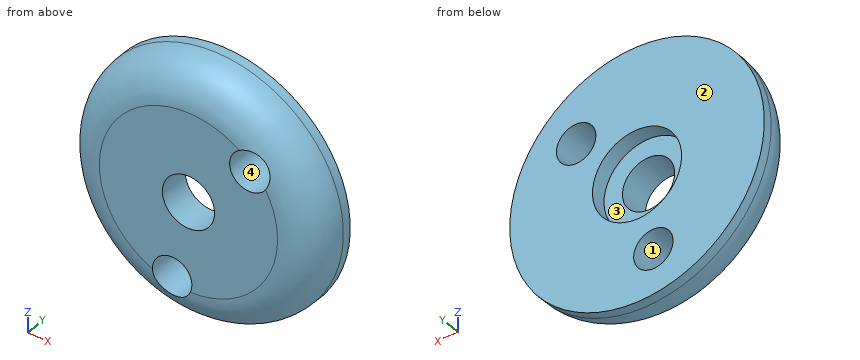
```python
from build123d import *

# Parameters (mm, degrees)
BOSS_EXTRUDE1_DEPTH        = 3
BOSS_EXTRUDE1_DEPTH_BACK   = 10
SKETCH1_R                  = 10
SKETCH4_R                  = 1.5
HOLE_DEPTH                 = 20.973741561
HOLECIR_COUNT              = 5
SKETCH6_R                  = 3.5
BEARINGHOLE_DEPTH          = 2.5
SKETCH7_R                  = 2.05
SHAFTHOLE_DEPTH            = 17.248076982
F_3_1_3_1_DIAMETER_HOLE1_D = 3.1
FILLET2_R                  = 3
SKETCH11_R                 = 10
CUT_EXTRUDE1_DEPTH         = 10


with BuildPart() as part:
    # Sketch1 → Boss-Extrude1 (new, two sides: drawn at the far end of the back side and taken through both)
    with BuildSketch(Plane(origin=(0, 0, 0), x_dir=(1, 0, 0), z_dir=(0, 1, 0)).offset(-BOSS_EXTRUDE1_DEPTH_BACK)):
        with Locations(Location((0, 0, 0), (0, 0, 270))):
            Circle(SKETCH1_R)
    extrude(amount=BOSS_EXTRUDE1_DEPTH + BOSS_EXTRUDE1_DEPTH_BACK)

    # Sketch4 → hole (cut, through all)
    with BuildSketch(Plane(origin=(-3.352872105, -1.093066116, 1.887711608), x_dir=(-0.4486862613641547, -0.14627571033740308, -0.8816371449912632), z_dir=(0.8382180262940947, 0.2732665289126682, -0.47192790187872385))):
        with Locations(Location((0, 0, 0), (0, 0, 8.746528197))):
            Circle(SKETCH4_R)
    hole = extrude(amount=-HOLE_DEPTH, mode=Mode.SUBTRACT)

    # holecir: hole ×5 about axis
    holecir_axis = Axis((0, 0, 0), (0, 1, 0))
    for i in range(1, HOLECIR_COUNT):
        add(hole.rotate(holecir_axis, i * 360 / HOLECIR_COUNT), mode=Mode.SUBTRACT)

    # Sketch6 → bearinghole (cut)
    with BuildSketch(Plane(origin=(0, -5, 0), x_dir=(-1, 0, 0), z_dir=(0, -1, 0))):
        with Locations(Location((0, 0, 0), (0, 0, 90))):
            Circle(SKETCH6_R)
    extrude(amount=BEARINGHOLE_DEPTH, mode=Mode.SUBTRACT)

    # Sketch7 → shafthole (cut, through all)
    with BuildSketch(Plane(origin=(0, -5, 0), x_dir=(-1, 0, 0), z_dir=(0, -1, 0))):
        with Locations(Location((0, 0, 0), (0, 0, 90))):
            Circle(SKETCH7_R)
    extrude(amount=SHAFTHOLE_DEPTH, mode=Mode.SUBTRACT)

    # Ø3.1 (3.1) Diameter Hole1 (through all)
    with Locations(Plane(origin=(0, 3, 0), x_dir=(1, 0, 0), z_dir=(0, 1, 0))):
        with Locations((-1.282558474, 6.372208703), (4.783101903, -4.401356176)):
            Hole(F_3_1_3_1_DIAMETER_HOLE1_D / 2)

    # Fillet2
    # the kernel refuses this fillet: 3 mm, written as the material it takes off along each edge
    with BuildSketch(Plane(origin=(0, 3, 0), x_dir=(0, 0, 1), z_dir=(-1, 0, 0))) as fillet2_piece_1:
        with BuildLine():
            CenterArc((10 - FILLET2_R, -FILLET2_R), FILLET2_R, 0, 90)
            Line((10 - FILLET2_R, 0), (10, 0))
            Line((10, 0), (10, -FILLET2_R))
        make_face()
    revolve(axis=Axis((0, 3, 0), (0, 1, 0)), mode=Mode.SUBTRACT)
    with BuildSketch(Plane(origin=(0, -10, 0), x_dir=(0, 0, 1), z_dir=(-1, 0, 0))) as fillet2_piece_2:
        with BuildLine():
            CenterArc((10 - FILLET2_R, FILLET2_R), FILLET2_R, 270, 90)
            Line((10 - FILLET2_R, 0), (10, 0))
            Line((10, 0), (10, FILLET2_R))
        make_face()
    revolve(axis=Axis((0, -10, 0), (0, 1, 0)), mode=Mode.SUBTRACT)

    # Sketch11 → Cut-Extrude1 (cut)
    with BuildSketch(Plane(origin=(0, -6.25, 0), x_dir=(-1, 0, 0), z_dir=(0, -1, 0))):
        with Locations(Location((0, 0, 0), (0, 0, 270))):
            Circle(SKETCH11_R)
    extrude(amount=-CUT_EXTRUDE1_DEPTH, mode=Mode.SUBTRACT)


solid = part.part
```
Can you work these out from the model? Positions are in its coordinate system, mm. Face numbers are marked on the shaded views. A direction names the side the tool comes from. Round coordinates to 2 decimals unless told otherwise and drop trailing zeros. Loops run counter-clockwise (first coordinate to the right, second up) from the corner with the lowest first, then second, coordinate; pieces in that order, holes last. Notation, with made-up numbers: (39.5, 38) -> (89.5, 38) arc R29 ccw to (89.5, 64) -> close; hole circle Ø1 at (83, -15). An arc over 180 degrees is marked (long way). One line per item, written item: value. Start each with the question number.
1. If we section it at B-B, the plane x = -1.5: Give the number of separate pieces and of enclosed holes in the cut face, then the cut area to 3 significant figures.
2. If we section it at C-C, the plane y = -7.85: Write out the boundary of the cut face in (x, z).
3. For the marked faces 3 and 4, which set-ups out of +Z, -Z, +X, -X, +Y, -Y let a thin tool reach every point of the face, with its end or its side?
4. If we section it at A-A, the plane y = -9.55: Write out the boundary of the cut face in (x, z).
5. If I drill on probe 1 along Z at (x, y) = (0, -8.6); probe 2 along Z at (x, y) = (0, -9.3); probe 3 along Y at (x, z) = (2.25, 0.75), over which ranges is the centre line in solid material (lowest first)?
6. If we mould it in two halves opening along Z, with no side actions, what happens to the marked faces 1 and 2? For each: pulls with the +Z half, pulls with the -Z half, needs draft (parallel to the pull), parting line crosses it, or undercut.
7. For pin 1 (2 mm diameter, centred on y = -9.5, z = 5.5, fed in from +X); pin 2 (10 mm diameter, centred on x = -6.5, z = -8, fed in from +Y); pin 3 (1.5 mm diameter, centred on y = -7, z = -2, fed in from +X), each with a flat end and sliding along its axis, tell me the tip position at first contact or that it passes through.
Calculated:
1. separate pieces: 3
1. enclosed holes: 0
1. area: 43.9 mm²
2. outline: circle Ø19.75 at (0, 0); hole circle Ø3.1 at (-1.28, -6.37); hole circle Ø4.1 at (0, 0); hole circle Ø3.1 at (4.78, 4.4)
3. face 3: +Y
3. face 4: +Y, -Y
4. outline: circle Ø17.16 at (0, 0); hole circle Ø3.1 at (-1.28, -6.37); hole circle Ø4.1 at (0, 0); hole circle Ø3.1 at (4.78, 4.4)
5. probe 1: z = -9.54 to -7.24, -5.5 to -2.05, 2.05 to 9.54
5. probe 2: z = -8.93 to -7.24, -5.5 to -2.05, 2.05 to 8.93
5. probe 3: y = -10 to -7.5
6. face 1: undercut
6. face 2: needs draft
7. pin 1: stops at x = 8.11
7. pin 2: stops at y = -6.25
7. pin 3: stops at x = 9.92
